The listing builds one solid part. Answer for the finished solid, in the listing's coordinates (mm). A direction names the side the tool comes from. Give positions to 0.01 mm unless a question says otherwise; leave off trailing zeros. Write each loop counter-clockwise with the first axis right and the second up, starting at its lowest first coordinate (ties: lowest second). Pieces come first, ordered by that corner, then holes. Notation, with made-up numbers: M 14.5,71 L 28.5,71 A4 cw 28.5,76 Z; hole C 63.25,55.25 d4. An arc over 180 degrees is marked long. Answer as a JSON object with one key per item and string values.
```python
from build123d import *

# Parameters (mm, degrees)
SKETCH1_W               = 40
SKETCH1_H               = 105
BOSS_EXTRUDE3_DEPTH     = 75
SKETCH4_W               = 97
SKETCH4_H               = 71
CUT_EXTRUDE2_DEPTH      = 36
SKETCH5_W               = 40
SKETCH5_H               = 9.8
CUT_EXTRUDE3_DEPTH      = 2
SKETCH6_W               = 40
SKETCH6_H               = 9.8
CUT_EXTRUDE4_DEPTH      = 2
SKETCH7_W               = 101
SKETCH7_H               = 9.8
CUT_EXTRUDE5_DEPTH      = 2
SKETCH8_R               = 1.55
CUT_EXTRUDE6_DEPTH      = 102
CUT_EXTRUDE6_DEPTH_BACK = 5
SKETCH9_W               = 8
SKETCH9_H               = 10
CUT_EXTRUDE7_DEPTH      = 2
SKETCH10_R              = 1.55
CUT_EXTRUDE8_DEPTH      = 2
SKETCH11_W              = 8
SKETCH11_H              = 10
CUT_EXTRUDE9_DEPTH      = 2
CUT_EXTRUDE10_REACH     = 42
SKETCH12_W              = 76
SKETCH12_H              = 55


with BuildPart() as part:
    # Sketch1 → Boss-Extrude3 (new body)
    with BuildSketch(Plane(origin=(0, 0, 0), x_dir=(1, 0, 0), z_dir=(0, 1, 0))):
        Rectangle(SKETCH1_W, SKETCH1_H)
    extrude(amount=BOSS_EXTRUDE3_DEPTH)

    # Sketch4 → Cut-Extrude2 (cut)
    with BuildSketch(Plane(origin=(20, 0, 0), x_dir=(0, 0, -1), z_dir=(1, 0, 0))):
        with Locations((0, 39.5)):
            Rectangle(SKETCH4_W, SKETCH4_H)
    extrude(amount=-CUT_EXTRUDE2_DEPTH, mode=Mode.SUBTRACT)

    # Sketch5 → Cut-Extrude3 (cut)
    with BuildSketch(Plane.XY.offset(52.5)):
        with Locations((0, 70.1)):
            Rectangle(SKETCH5_W, SKETCH5_H)
    extrude(amount=-CUT_EXTRUDE3_DEPTH, mode=Mode.SUBTRACT)

    # Sketch6 → Cut-Extrude4 (cut)
    with BuildSketch(Plane(origin=(0, 0, -52.5), x_dir=(-1, 0, 0), z_dir=(0, 0, -1))):
        with Locations((0, 70.1)):
            Rectangle(SKETCH6_W, SKETCH6_H)
    extrude(amount=-CUT_EXTRUDE4_DEPTH, mode=Mode.SUBTRACT)

    # Sketch7 → Cut-Extrude5 (cut)
    with BuildSketch(Plane.ZY.offset(20)):
        with Locations((0, 70.1)):
            Rectangle(SKETCH7_W, SKETCH7_H)
    extrude(amount=-CUT_EXTRUDE5_DEPTH, mode=Mode.SUBTRACT)

    # Sketch8 → Cut-Extrude6 (cut, two sides)
    with BuildSketch(Plane(origin=(0, 0, 48.5), x_dir=(-1, 0, 0), z_dir=(0, 0, -1))) as cut_extrude6_sk:
        with Locations((-16, 18)):
            Circle(SKETCH8_R)
        with Locations((-16, 46)):
            Circle(SKETCH8_R)
    extrude(amount=CUT_EXTRUDE6_DEPTH, mode=Mode.SUBTRACT)
    extrude(cut_extrude6_sk.sketch, amount=-CUT_EXTRUDE6_DEPTH_BACK, mode=Mode.SUBTRACT)

    # Sketch9 → Cut-Extrude7 (cut)
    with BuildSketch(Plane(origin=(0, 0, 48.5), x_dir=(-1, 0, 0), z_dir=(0, 0, -1))):
        with Locations((-16, 18)):
            Rectangle(SKETCH9_W, SKETCH9_H)
        with Locations((-16, 46)):
            Rectangle(SKETCH9_W, SKETCH9_H)
    extrude(amount=-CUT_EXTRUDE7_DEPTH, mode=Mode.SUBTRACT)

    # Sketch10 → Cut-Extrude8 (cut)
    with BuildSketch(Plane.ZY.offset(18)):
        with Locations((0, 71)):
            Circle(SKETCH10_R)
    extrude(amount=-CUT_EXTRUDE8_DEPTH, mode=Mode.SUBTRACT)

    # Sketch11 → Cut-Extrude9 (cut)
    with BuildSketch(Plane.XY.offset(-48.5)):
        with Locations((16, 46)):
            Rectangle(SKETCH11_W, SKETCH11_H)
        with Locations((16, 18)):
            Rectangle(SKETCH11_W, SKETCH11_H)
    extrude(amount=-CUT_EXTRUDE9_DEPTH, mode=Mode.SUBTRACT)

    # Sketch12 → Cut-Extrude10 (cut, up to next)
    with BuildSketch(Plane.ZY.offset(20), mode=Mode.PRIVATE) as cut_extrude10_sk1:
        with Locations((0, 33.5)):
            Rectangle(SKETCH12_W, SKETCH12_H)
    cut_extrude10_tool1 = extrude(cut_extrude10_sk1.sketch, amount=-CUT_EXTRUDE10_REACH, mode=Mode.PRIVATE) & part.part
    add(cut_extrude10_tool1.solids().sort_by_distance((-20, 33.5, 0))[0], mode=Mode.SUBTRACT)


solid = part.part
```
1. A cutting plane is placed at B-B, the plane z = 0. Give the vertices of the cut face in (x, y).
Verdict:
{"outline": "M -20,0 L 20,0 L 20,4 L -16,4 L -16,6 L -20,6 Z; M -20,61 L -16,61 L -16,69.45 L -18,69.45 L -18,65.2 L -20,65.2 Z; M -18,72.55 L -16,72.55 L -16,75 L -18,75 Z"}
2. A cutting plane is placed at D-D, the plane z = -45. Give the vertices of the cut face in (x, y), plus the area to 3 significant figures.
Verdict:
{"outline": "M -20,0 L 20,0 L 20,4 L -16,4 L -16,75 L -18,75 L -18,65.2 L -20,65.2 Z", "area": "424 mm2"}
3. For faces 1 (the flat face through (-20, 3, 1)), 2 (the flat face through (14, 18, 50.5)), 3 (the flat face through (-16, 64, 1)), 4 (the flat face through (-18, 61, -1)), 5 (the flat face through (1, 70, 50.5)), determine the directions among +Z, -Z, +X, -X, +Y, -Y from which every point of the face is accessible in a straight line to the end or side of a thin tool.
Verdict:
{"face 1": "+Z, -Z, -X, +Y, -Y", "face 2": "+X", "face 3": "+X, +Y", "face 4": "+X, -X", "face 5": "+Z, +X, -X, +Y"}
4. The mould has two halves that part along Z. Classify faces 6 (the flat face through (-18, 69, -1)), 7 (the flat face through (14, 46, 50.5)), 8 (the flat face through (18, 46, -50.5)), 9 (the flat face through (0, 32, 52.5)): released by +Z, released by -Z, zero draft, split by the parting line, or undercut.
Verdict:
{"face 6": "zero draft", "face 7": "undercut", "face 8": "undercut", "face 9": "released by +Z"}
5. Flat-ended cylindrical pins translate along their axes: pin 1 (3 mm diameter, centred on y = 68, z = 7, fed in from -X); pin 2 (2 mm diameter, centred on y = 45.5, z = -49, fed in from +X); pin 3 (20 mm diameter, centred on x = 7, z = 25, fed in from +Y). Find the tip coordinate at first contact, or state that the pin passes through.
Verdict:
{"pin 1": "stops at x = -18", "pin 2": "stops at x = 12", "pin 3": "stops at y = 4"}
6. A cutting plane is placed at A-A, the plane y = 18. Give the vertices of the cut face in (x, z).
Verdict:
{"outline": "M -20,-52.5 L 14.45,-52.5 L 14.45,-50.5 L 12,-50.5 L 12,-48.5 L -16,-48.5 L -16,-38 L -20,-38 Z; M -20,38 L -16,38 L -16,48.5 L 12,48.5 L 12,50.5 L 14.45,50.5 L 14.45,52.5 L -20,52.5 Z; M 17.55,-52.5 L 20,-52.5 L 20,-50.5 L 17.55,-50.5 Z; M 17.55,50.5 L 20,50.5 L 20,52.5 L 17.55,52.5 Z"}
7. A cutting plane is placed at C-C, the plane y = 33.5. Give the vertices of the cut face in (x, z).
Verdict:
{"outline": "M -20,-52.5 L 20,-52.5 L 20,-48.5 L -16,-48.5 L -16,-38 L -20,-38 Z; M -20,38 L -16,38 L -16,48.5 L 20,48.5 L 20,52.5 L -20,52.5 Z"}
8. Consider line 1 along Y through (x, z) = (16, -51); line 2 along Y through (x, z) = (-17, 0); line 3 along Z through (x, y) = (-4, 53). Determine where each line is inside the solid, lowest interval first.
Verdict:
{"line 1": "y = 0 to 16.45, 19.55 to 44.45, 47.55 to 65.2", "line 2": "y = 0 to 6, 61 to 69.45, 72.55 to 75", "line 3": "z = -52.5 to -48.5, 48.5 to 52.5"}
